Can you work these out from the model? Positions are in its coordinate system, mm. Give positions to 0.01 mm unless a question says otherwise; leave off trailing zeros. Write each loop counter-clockwise with the first axis right and the second up, starting at its lowest first coordinate (ties: lowest second). Pieces come first, ordered by that corner, then holes.
1. I'm going to push flat-ended pins straight in: pin 1 (1.1 mm diameter, centred on x = -0.5, z = -363.5, fed in from -Y); pin 2 (2 mm diameter, centred on y = 2.5, z = -300.5, fed in from +X); pin 3 (0.5 mm diameter, centred on x = -17, z = -347, fed in from +Y). Where does each tip first touch, or does it pass through?
2. If I drill on probe 1 along Y at (x, z) = (-6.5, -315); probe 2 along Y at (x, z) = (0, -379); probe 3 along X at (y, z) = (-5, -410), over which ranges is the centre line in solid material (lowest first)?
3. Suppose I cut it at A-A (x = 0). Please give me the cut outline in (y, z), and give its area (3 significant figures).
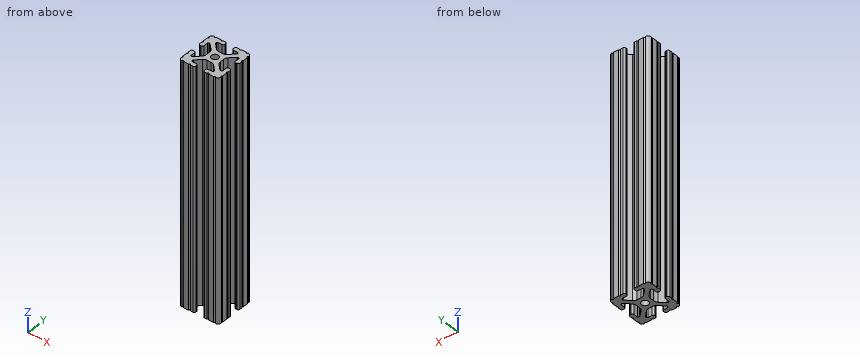
```python
from build123d import *

# Parameters (mm, degrees)
SKETCH3_R                = 3.3274
BOSS_EXTRUDE1_DEPTH      = 457.2
BOSS_EXTRUDE1_DEPTH_BACK = 457.2
CUT_EXTRUDE1_DEPTH       = 22.86


with BuildPart() as part:
    # Sketch3 → Boss-Extrude1 (new body, two sides)
    with BuildSketch(Plane.XY) as boss_extrude1_sk:
        with BuildLine():
            Line((-4.064, 16.539617549), (-4.064, 17.496382451))
            ThreePointArc((-4.064, 17.496382451), (-4.519044045, 18.594955955), (-5.617617549, 19.05))
            Line((-5.617617549, 19.05), (-7.974178704, 19.05))
            ThreePointArc((-7.974178704, 19.05), (-8.736178704, 18.288), (-9.498178704, 19.05))
            Line((-9.498178704, 19.05), (-14.327719207, 19.05))
            ThreePointArc((-14.327719207, 19.05), (-15.087603123, 18.231251131), (-15.847487039, 19.05))
            ThreePointArc((-15.847487039, 19.05), (-18.120176289, 18.120192083), (-19.05, 15.847509295))
            ThreePointArc((-19.05, 15.847509295), (-18.231250992, 15.08762539), (-19.05, 14.327741484))
            Line((-19.05, 14.327741484), (-19.05, 9.496091471))
            ThreePointArc((-19.05, 9.496091471), (-18.231250992, 8.736207565), (-19.05, 7.97632366))
            Line((-19.05, 7.97632366), (-19.05, 5.617617549))
            ThreePointArc((-19.05, 5.617617549), (-18.594955955, 4.519044045), (-17.496382451, 4.064))
            Line((-17.496382451, 4.064), (-16.539617549, 4.064))
            ThreePointArc((-16.539617549, 4.064), (-15.441044045, 4.519044045), (-14.986, 5.617617549))
            Line((-14.986, 5.617617549), (-14.986, 9.385342516))
            ThreePointArc((-14.986, 9.385342516), (-14.721898185, 10.022940701), (-14.0843, 10.287042516))
            Line((-14.0843, 10.287042516), (-13.516042086, 10.287042516))
            ThreePointArc((-13.516042086, 10.287042516), (-13.170975923, 10.218404478), (-12.878443117, 10.022939917))
            Line((-12.878443117, 10.022939917), (-8.14758008, 5.292065243))
            ThreePointArc((-8.14758008, 5.292065243), (-7.117955879, 3.751120653), (-6.7564, 1.933453584))
            Line((-6.7564, 1.933453584), (-6.7564, -1.933453584))
            ThreePointArc((-6.7564, -1.933453584), (-7.117955879, -3.751120653), (-8.14758008, -5.292065243))
            Line((-8.14758008, -5.292065243), (-12.878443117, -10.022939917))
            ThreePointArc((-12.878443117, -10.022939917), (-13.170975923, -10.218404478), (-13.516042086, -10.287042516))
            Line((-13.516042086, -10.287042516), (-14.0843, -10.287042516))
            ThreePointArc((-14.0843, -10.287042516), (-14.721898185, -10.022940701), (-14.986, -9.385342516))
            Line((-14.986, -9.385342516), (-14.986, -5.617617549))
            ThreePointArc((-14.986, -5.617617549), (-15.441044045, -4.519044045), (-16.539617549, -4.064))
            Line((-16.539617549, -4.064), (-17.496382451, -4.064))
            ThreePointArc((-17.496382451, -4.064), (-18.594955955, -4.519044045), (-19.05, -5.617617549))
            Line((-19.05, -5.617617549), (-19.05, -7.976318491))
            ThreePointArc((-19.05, -7.976318491), (-18.231250992, -8.736202396), (-19.05, -9.496086302))
            Line((-19.05, -9.496086302), (-19.05, -14.32774291))
            ThreePointArc((-19.05, -14.32774291), (-18.231250992, -15.087626816), (-19.05, -15.847510721))
            ThreePointArc((-19.05, -15.847510721), (-18.120175716, -18.120192644), (-15.847486868, -19.05))
            ThreePointArc((-15.847486868, -19.05), (-15.087602952, -18.231251131), (-14.327719036, -19.05))
            Line((-14.327719036, -19.05), (-9.496062448, -19.05))
            ThreePointArc((-9.496062448, -19.05), (-8.736178532, -18.231251131), (-7.976294616, -19.05))
            Line((-7.976294616, -19.05), (-5.617617549, -19.05))
            ThreePointArc((-5.617617549, -19.05), (-4.519044045, -18.594955955), (-4.064, -17.496382451))
            Line((-4.064, -17.496382451), (-4.064, -16.539617549))
            ThreePointArc((-4.064, -16.539617549), (-4.519044045, -15.441044045), (-5.617617549, -14.986))
            Line((-5.617617549, -14.986), (-9.3853, -14.986))
            ThreePointArc((-9.3853, -14.986), (-10.022898185, -14.721898185), (-10.287, -14.0843))
            Line((-10.287, -14.0843), (-10.287, -13.552357131))
            ThreePointArc((-10.287, -13.552357131), (-10.218362387, -13.207291992), (-10.022898969, -12.91475973))
            Line((-10.022898969, -12.91475973), (-5.252158105, -8.144007132))
            ThreePointArc((-5.252158105, -8.144007132), (-3.715177372, -7.117027388), (-1.902183975, -6.7564))
            Line((-1.902183975, -6.7564), (1.902183975, -6.7564))
            ThreePointArc((1.902183975, -6.7564), (3.715177372, -7.117027388), (5.252158105, -8.144007132))
            Line((5.252158105, -8.144007132), (10.022898969, -12.91475973))
            ThreePointArc((10.022898969, -12.91475973), (10.218362387, -13.207291992), (10.287, -13.552357131))
            Line((10.287, -13.552357131), (10.287, -14.0843))
            ThreePointArc((10.287, -14.0843), (10.022898185, -14.721898185), (9.3853, -14.986))
            Line((9.3853, -14.986), (5.617617549, -14.986))
            ThreePointArc((5.617617549, -14.986), (4.519044045, -15.441044045), (4.064, -16.539617549))
            Line((4.064, -16.539617549), (4.064, -17.496382451))
            ThreePointArc((4.064, -17.496382451), (4.519044045, -18.594955955), (5.617617549, -19.05))
            Line((5.617617549, -19.05), (7.976294616, -19.05))
            ThreePointArc((7.976294616, -19.05), (8.736178532, -18.231251131), (9.496062448, -19.05))
            Line((9.496062448, -19.05), (14.327719036, -19.05))
            ThreePointArc((14.327719036, -19.05), (15.087602952, -18.231251131), (15.847486868, -19.05))
            ThreePointArc((15.847486868, -19.05), (18.120175716, -18.120192644), (19.05, -15.847510721))
            ThreePointArc((19.05, -15.847510721), (18.231250992, -15.087626816), (19.05, -14.32774291))
            Line((19.05, -14.32774291), (19.05, -9.496086302))
            ThreePointArc((19.05, -9.496086302), (18.231250992, -8.736202396), (19.05, -7.976318491))
            Line((19.05, -7.976318491), (19.05, -5.617617549))
            ThreePointArc((19.05, -5.617617549), (18.594955955, -4.519044045), (17.496382451, -4.064))
            Line((17.496382451, -4.064), (16.539617549, -4.064))
            ThreePointArc((16.539617549, -4.064), (15.441044045, -4.519044045), (14.986, -5.617617549))
            Line((14.986, -5.617617549), (14.986, -9.385342516))
            ThreePointArc((14.986, -9.385342516), (14.721898185, -10.022940701), (14.0843, -10.287042516))
            Line((14.0843, -10.287042516), (13.516042086, -10.287042516))
            ThreePointArc((13.516042086, -10.287042516), (13.170975923, -10.218404478), (12.878443117, -10.022939917))
            Line((12.878443117, -10.022939917), (8.14758008, -5.292065243))
            ThreePointArc((8.14758008, -5.292065243), (7.117955879, -3.751120653), (6.7564, -1.933453584))
            Line((6.7564, -1.933453584), (6.7564, 1.933453584))
            ThreePointArc((6.7564, 1.933453584), (7.117955879, 3.751120653), (8.14758008, 5.292065243))
            Line((8.14758008, 5.292065243), (12.878443117, 10.022939917))
            ThreePointArc((12.878443117, 10.022939917), (13.170975923, 10.218404478), (13.516042086, 10.287042516))
            Line((13.516042086, 10.287042516), (14.0843, 10.287042516))
            ThreePointArc((14.0843, 10.287042516), (14.721898185, 10.022940701), (14.986, 9.385342516))
            Line((14.986, 9.385342516), (14.986, 5.617617549))
            ThreePointArc((14.986, 5.617617549), (15.441044045, 4.519044045), (16.539617549, 4.064))
            Line((16.539617549, 4.064), (17.496382451, 4.064))
            ThreePointArc((17.496382451, 4.064), (18.594955955, 4.519044045), (19.05, 5.617617549))
            Line((19.05, 5.617617549), (19.05, 7.97632366))
            ThreePointArc((19.05, 7.97632366), (18.231250992, 8.736207565), (19.05, 9.496091471))
            Line((19.05, 9.496091471), (19.05, 14.327741484))
            ThreePointArc((19.05, 14.327741484), (18.231250992, 15.08762539), (19.05, 15.847509295))
            ThreePointArc((19.05, 15.847509295), (18.120176289, 18.120192083), (15.847487039, 19.05))
            ThreePointArc((15.847487039, 19.05), (15.087603123, 18.231251131), (14.327719207, 19.05))
            Line((14.327719207, 19.05), (9.498178704, 19.05))
            ThreePointArc((9.498178704, 19.05), (8.736178704, 18.288), (7.974178704, 19.05))
            Line((7.974178704, 19.05), (5.617617549, 19.05))
            ThreePointArc((5.617617549, 19.05), (4.519044045, 18.594955955), (4.064, 17.496382451))
            Line((4.064, 17.496382451), (4.064, 16.539617549))
            ThreePointArc((4.064, 16.539617549), (4.519044045, 15.441044045), (5.617617549, 14.986))
            Line((5.617617549, 14.986), (9.3853, 14.986))
            ThreePointArc((9.3853, 14.986), (10.022898185, 14.721898185), (10.287, 14.0843))
            Line((10.287, 14.0843), (10.287, 13.552357131))
            ThreePointArc((10.287, 13.552357131), (10.218362387, 13.207291992), (10.022898969, 12.91475973))
            Line((10.022898969, 12.91475973), (5.252158105, 8.144007132))
            ThreePointArc((5.252158105, 8.144007132), (3.715177372, 7.117027388), (1.902183975, 6.7564))
            Line((1.902183975, 6.7564), (-1.902183975, 6.7564))
            ThreePointArc((-1.902183975, 6.7564), (-3.715177372, 7.117027388), (-5.252158105, 8.144007132))
            Line((-5.252158105, 8.144007132), (-10.022898969, 12.91475973))
            ThreePointArc((-10.022898969, 12.91475973), (-10.218362387, 13.207291992), (-10.287, 13.552357131))
            Line((-10.287, 13.552357131), (-10.287, 14.0843))
            ThreePointArc((-10.287, 14.0843), (-10.022898185, 14.721898185), (-9.3853, 14.986))
            Line((-9.3853, 14.986), (-5.617617549, 14.986))
            ThreePointArc((-5.617617549, 14.986), (-4.519044045, 15.441044045), (-4.064, 16.539617549))
        make_face()
        Circle(SKETCH3_R, mode=Mode.SUBTRACT)
    extrude(amount=BOSS_EXTRUDE1_DEPTH)
    extrude(boss_extrude1_sk.sketch, amount=-BOSS_EXTRUDE1_DEPTH_BACK)

    # Sketch4 → Cut-Extrude1 (cut, symmetric)
    with BuildSketch(Plane(origin=(0, 0, 0), x_dir=(1, 0, 0), z_dir=(0, 1, 0))):
        Polygon((-11.912948955, 228.6), (-26.025980117, 228.6), (-26.025980117, -478.373467622), (32.635256624, -478.373467622), (32.635256624, 228.6), align=None)
    extrude(amount=CUT_EXTRUDE1_DEPTH, both=True, mode=Mode.SUBTRACT)


solid = part.part
```
Checks:
1. pin 1: stops at y = -6.76
1. pin 2: stops at x = 7.02
1. pin 3: stops at y = 18.93
2. probe 1: y = -19.05 to -14.99, -9.39 to 9.39, 14.99 to 19.05
2. probe 2: y = -6.76 to -3.33, 3.33 to 6.76
2. probe 3: x = -18.92 to -15.11, -7.88 to 7.88, 15.11 to 18.92
3. outline: (-6.76, -457.2) - (-3.33, -457.2) - (-3.33, -228.6) - (-6.76, -228.6) - close; (3.33, -457.2) - (6.76, -457.2) - (6.76, -228.6) - (3.33, -228.6) - close
3. area: 1,570 mm2
